Here's how the part is built. I have some questions about the finished solid (model axes, mm). A direction names the side the tool comes from. Round coordinates to 2 decimals unless told otherwise and drop trailing zeros. Write each loop counter-clockwise with the first axis right and the second up, starting at its lowest first coordinate (ties: lowest second). Pieces come first, ordered by that corner, then holes. Notation, with made-up numbers: (-23.75, 61) -> (2.25, 61) arc R37 cw to (2.25, 98) -> close; hole circle Ø7 at (48, 25.5). An arc over 180 degrees is marked (long way). Answer as CSV lines item,"result".
from build123d import *

# Parameters (mm, degrees)
SKETCH_5_W          = 60
SKETCH_5_H          = 115
EXTRUDE_2_DEPTH     = 20
SKETCH_1_R          = 1.3
CUT_EXTRUDE_4_DEPTH = 20
SKETCH_6_R          = 5
EXTRUDE_3_DEPTH     = 13
SKETCH_22_R         = 9.5
CUT_EXTRUDE_5_DEPTH = 15
SKETCH_22_10_R      = 9.5
CUT_EXTRUDE_6_DEPTH = 15


with BuildPart() as part:
    # Sketch 5 → Extrude 2 (new body)
    with BuildSketch(Plane.XY):
        with Locations((85.095319229, -3)):
            Rectangle(SKETCH_5_W, SKETCH_5_H)
    extrude(amount=EXTRUDE_2_DEPTH)

    # Sketch 1 → Cut-Extrude 4 (cut)
    with BuildSketch(Plane.XY):
        with Locations((59.19, 1.7)):
            Circle(SKETCH_1_R)
        with Locations((106.81, 1.7)):
            Circle(SKETCH_1_R)
        with Locations((106.81, -7.7)):
            Circle(SKETCH_1_R)
        with Locations((59.19, -7.7)):
            Circle(SKETCH_1_R)
        Polygon((55, -3), (55, 0), (62, 0), (62, 7.5), (104, 7.5), (104, -13.5), (62, -13.5), (62, -6), (55, -6), align=None)
    extrude(amount=CUT_EXTRUDE_4_DEPTH, mode=Mode.SUBTRACT)

    # Sketch 6 → Extrude 3 (add)
    with BuildSketch(Plane(origin=(115, 0, 0), x_dir=(0, 0, -1), z_dir=(1, 0, 0))):
        with Locations((-10, 44.5)):
            Circle(SKETCH_6_R)
        with Locations((-10, 29.5)):
            Circle(SKETCH_6_R)
        with Locations((-10, -35.5)):
            Circle(SKETCH_6_R)
        with Locations((-10, -50.5)):
            Circle(SKETCH_6_R)
    extrude(amount=EXTRUDE_3_DEPTH)

    # Sketch 22 → Cut-Extrude 5 (cut)
    with BuildSketch(Plane.XY):
        with Locations((85, 37.5)):
            Circle(SKETCH_22_R)
    extrude(amount=CUT_EXTRUDE_5_DEPTH, mode=Mode.SUBTRACT)

    # Sketch 22_10 → Cut-Extrude 6 (cut)
    with BuildSketch(Plane.XY):
        with Locations((85, -43.5)):
            Circle(SKETCH_22_10_R)
    extrude(amount=CUT_EXTRUDE_6_DEPTH, mode=Mode.SUBTRACT)


solid = part.part
Item 1: If we mould it in two halves opening along X, with no side actions, what happens to faces 1 (the flat face through (128, -35, 10)), 2 (the flat face through (83, -13.5, 10)), 3 (the flat face through (85, 11, 0)), 4 (the flat face through (55.095, -34, 10))? For each: pulls with the +X half, pulls with the -X half, needs draft (parallel to the pull), parting line crosses it, or undercut.
Results found:
face 1,"pulls with the +X half"
face 2,"undercut"
face 3,"needs draft"
face 4,"pulls with the -X half"
Item 2: Will these pins go through, and if not, where does the flat tip stop? pin 1 (6 mm diameter, centred on y = 3, z = 9, fed in from +X); pin 2 (4 mm diameter, centred on x = 106.81, y = 1.7, fed in from -Z); pin 3 (5.5 mm diameter, centred on x = 87, y = 34, fed in from -Z); pin 4 (1 mm diameter, centred on x = 118, y = 34.5, fed in from -Z).
Results found:
pin 1,"stops at x = 115.1"
pin 2,"stops at z = 0"
pin 3,"stops at z = 15"
pin 4,"stops at z = 7.82"
Item 3: For faces 5 (the flat face through (62, -10, 10)), 6 (the cylindrical face through (121.457, 27.585, 5.381)), 7 (the flat face through (59, -6, 10)), 8 (the flat face through (85, 11, 20)), 9 (the cylindrical face through (94.061, 40.354, 7.395)), which set-ups out of +Z, -Z, +X, -X, +Y, -Y let a thin tool reach every point of the face, with its end or its side?
Results found:
face 5,"+Z, -Z"
face 6,"+X"
face 7,"+Z, -Z, -X"
face 8,"+Z, +X, -X, +Y, -Y"
face 9,"-Z"
Item 4: Suppose I cut it at A-A, the plane x = 85. List the corners of the cut face in (y, z) for me, then the cut area to 3 significant figures.
Results found:
outline,"(-60.5, 0) -> (-53, 0) -> (-53, 15) -> (-34, 15) -> (-34, 0) -> (-13.5, 0) -> (-13.5, 20) -> (-60.5, 20) -> close; (7.5, 0) -> (28, 0) -> (28, 15) -> (47, 15) -> (47, 0) -> (54.5, 0) -> (54.5, 20) -> (7.5, 20) -> close"
area,"1,310 mm²"
Item 5: I need wall thicknesses on L1, parallel to Y at x = 59.19, z = 7.5; L2, parallel to Y at x = 85, z = 8.25; L3, parallel to Y at x = 106.81, z = 7.5. Which ranges of each line are inside material? Lowest first, please.
Results found:
L1,"y = -60.5 to -9, -6.4 to -6, 0 to 0.4, 3 to 54.5"
L2,"y = -60.5 to -53, -34 to -13.5, 7.5 to 28, 47 to 54.5"
L3,"y = -60.5 to -9, -6.4 to 0.4, 3 to 54.5"
Item 6: Suppose I cut it at D-D, the plane z = 18. List the corners of the cut face in (x, y) for me.
Results found:
outline,"(55.1, -60.5) -> (115.1, -60.5) -> (115.1, 54.5) -> (55.1, 54.5) -> (55.1, 0) -> (62, 0) -> (62, 7.5) -> (104, 7.5) -> (104, -13.5) -> (62, -13.5) -> (62, -6) -> (55.1, -6) -> close; hole circle Ø2.6 at (59.19, -7.7); hole circle Ø2.6 at (59.19, 1.7); hole circle Ø2.6 at (106.81, -7.7); hole circle Ø2.6 at (106.81, 1.7)"
Item 7: Suppose I cut it at B-B, the plane y = -7.7. List the corners of the cut face in (x, z) for me.
Results found:
outline,"(55.1, 0) -> (57.89, 0) -> (57.89, 20) -> (55.1, 20) -> close; (60.49, 0) -> (62, 0) -> (62, 20) -> (60.49, 20) -> close; (104, 0) -> (105.51, 0) -> (105.51, 20) -> (104, 20) -> close; (108.11, 0) -> (115.1, 0) -> (115.1, 20) -> (108.11, 20) -> close"
Item 8: Suppose I cut it at C-C, the plane x = 106.81. List the corners of the cut face in (y, z) for me, then the cut area to 3 significant figures.
Results found:
outline,"(-60.5, 0) -> (-9, 0) -> (-9, 20) -> (-60.5, 20) -> close; (-6.4, 0) -> (0.4, 0) -> (0.4, 20) -> (-6.4, 20) -> close; (3, 0) -> (54.5, 0) -> (54.5, 20) -> (3, 20) -> close"
area,"2,200 mm²"
